For this review, take the finished solid that the model builds, in its own axes (mm). A direction names the side the tool comes from. Coordinates: 2 decimals unless noted, no trailing zeros. Write each loop counter-clockwise with the first axis right and the second up, starting at its lowest first coordinate (ties: lowest second). Pieces come first, ordered by that corner, then holes. Notation, with made-up numbers: (-27.75, -20.5) -> (17.25, -20.5) arc R17 cw to (17.25, 5.5) -> close; hole circle Ø9 at (-4.5, 65). An arc over 180 degrees is marked (long way). Put each result on its own line as item: value. Start each with the question number.
Item 1: Consider section C-C on z = 5. Give the boundary of the cut face in (x, y), and give its area (3 significant figures).
Item 2: The part is to be moulded in two halves that separate along X. For faces 6 (the flat face through (-6, 3, 8)), 7 (the flat face through (0, 10.339, 4)), 8 (the cylindrical face through (8.916, 8.761, 3.944)), say which applies: +X half, -X half, draft (parallel to the pull), parting line (faces both ways), or undercut.
Item 3: Consider section B-B on x = 4.75. Give the boundary of the cut face in (y, z).
Item 4: For faces 1 (the flat face through (11, -2, 4)), 2 (the cylindrical face through (-8.916, -8.761, 3.944)), 3 (the flat face through (2, -11, 4)), 4 (the flat face through (-11, 2, 4)), 5 (the flat face through (-2, 11, 4)), list the 3-axis set-ups (+Z, -Z, +X, -X, +Y, -Y) from which the entire face can be reached by the end or side of a thin tool; tool diameter is ignored.
Item 5: Insertion check: P1, Ø1.6, axis at x = 11, z = 4.5, coming from the +Y side; P2, Ø4.5, axis at y = -0.5, z = 3, coming from the -X side; P3, Ø3, axis at y = 8, z = 6, coming from the -X side; P4, Ø7, axis at x = 0, y = 0, coming from the +Z side. Each pin has a flat end and moves straight along its axis. Give the tip position at first contact, or say it passes through.
Item 6: To check wall thickness, follow L1, parallel to Y at x = 0, z = 4.25; L2, parallel to X at y = 2.75, z = 1.75; L3, parallel to X at y = -4.5, z = 7.75. State the ranges of each line that lie inside material, in increasing order.
Item 7: Consider section D-D on y = -8.25. Give the boundary of the cut face in (x, z).
Item 8: Consider section A-A on y = 0. Give the boundary of the cut face in (x, z).
```python
from build123d import *

# Parameters (mm, degrees)
ESBO_O1_R                = 6
RESSALTO_EXTRUS_O1_DEPTH = 8


with BuildPart() as part:
    # Esboço1 → Ressalto-extrusão1 (new body)
    with BuildSketch(Plane.XY):
        with BuildLine():
            Line((2, 10.338962679), (-2, 10.338962679))
            Line((-2, 10.338962679), (-2, 12.338962679))
            ThreePointArc((-2, 12.338962679), (-8.838834765, 8.838834765), (-12.338962679, 2))
            Line((-12.338962679, 2), (-10.338962679, 2))
            Line((-10.338962679, 2), (-10.338962679, -2))
            Line((-10.338962679, -2), (-12.338962679, -2))
            ThreePointArc((-12.338962679, -2), (-8.838834765, -8.838834765), (-2, -12.338962679))
            Line((-2, -12.338962679), (-2, -10.338962679))
            Line((-2, -10.338962679), (2, -10.338962679))
            Line((2, -10.338962679), (2, -12.338962679))
            ThreePointArc((2, -12.338962679), (8.838834765, -8.838834765), (12.338962679, -2))
            Line((12.338962679, -2), (10.338962679, -2))
            Line((10.338962679, -2), (10.338962679, 2))
            Line((10.338962679, 2), (12.338962679, 2))
            ThreePointArc((12.338962679, 2), (8.838834765, 8.838834765), (2, 12.338962679))
            Line((2, 12.338962679), (2, 10.338962679))
        make_face()
        Circle(ESBO_O1_R, mode=Mode.SUBTRACT)
    extrude(amount=RESSALTO_EXTRUS_O1_DEPTH)


solid = part.part
```
Return value:
1. outline: (-12.34, -2) arc R12.5 ccw to (-2, -12.34) -> (-2, -10.34) -> (2, -10.34) -> (2, -12.34) arc R12.5 ccw to (12.34, -2) -> (10.34, -2) -> (10.34, 2) -> (12.34, 2) arc R12.5 ccw to (2, 12.34) -> (2, 10.34) -> (-2, 10.34) -> (-2, 12.34) arc R12.5 ccw to (-12.34, 2) -> (-10.34, 2) -> (-10.34, -2) -> close; hole circle Ø12 at (0, 0)
1. area: 344 mm^2
2. face 6: draft
2. face 7: undercut
2. face 8: +X half
3. outline: (-11.56, 0) -> (-3.67, 0) -> (-3.67, 8) -> (-11.56, 8) -> close; (3.67, 0) -> (11.56, 0) -> (11.56, 8) -> (3.67, 8) -> close
4. face 1: +Z, -Z, +X
4. face 2: +Z, -Z, -X, -Y
4. face 3: +Z, -Z, -Y
4. face 4: +Z, -Z, -X
4. face 5: +Z, -Z, +Y
5. P1: y = 7.23
5. P2: x = -12.34
5. P3: x = -10.68
5. P4: through
6. L1: -10.34 to -6, 6 to 10.34
6. L2: -12.19 to -5.33, 5.33 to 12.19
6. L3: -11.66 to -3.97, 3.97 to 11.66
7. outline: (-9.39, 0) -> (9.39, 0) -> (9.39, 8) -> (-9.39, 8) -> close
8. outline: (-10.34, 0) -> (-6, 0) -> (-6, 8) -> (-10.34, 8) -> close; (6, 0) -> (10.34, 0) -> (10.34, 8) -> (6, 8) -> close
